from build123d import *

# Parameters (mm, degrees)
SKETCH1_W           = 141.478
SKETCH1_H           = 121.412
SKETCH1_R           = 3.175
SKETCH1_W_2         = 98.298
SKETCH1_H_2         = 38.862
BOSS_EXTRUDE1_DEPTH = 6.35
SKETCH2_W           = 61.473578211
SKETCH2_H           = 35.56
CUT_EXTRUDE1_DEPTH  = 3.81
SKETCH3_R           = 1.143
CUT_EXTRUDE2_DEPTH  = 158.770193915
SKETCH4_R           = 1.905
CUT_EXTRUDE3_DEPTH  = 158.770193915


with BuildPart() as part:
    # Sketch1 → Boss-Extrude1 (new body)
    with BuildSketch(Plane.XY):
        with Locations((49.149, 41.656)):
            Rectangle(SKETCH1_W, SKETCH1_H)
        with Locations((98.298, 80.772)):
            Circle(SKETCH1_R, mode=Mode.SUBTRACT)
        with Locations((49.149, 19.431)):
            Rectangle(SKETCH1_W_2, SKETCH1_H_2, mode=Mode.SUBTRACT)
    extrude(amount=BOSS_EXTRUDE1_DEPTH)

    # Sketch2 → Cut-Extrude1 (cut)
    with BuildSketch(Plane(origin=(0, 0, 0), x_dir=(-1, 0, 0), z_dir=(0, 0, -1))):
        with Locations((-30.736789106, 56.642)):
            Rectangle(SKETCH2_W, SKETCH2_H)
    extrude(amount=-CUT_EXTRUDE1_DEPTH, mode=Mode.SUBTRACT)

    # Sketch3 → Cut-Extrude2 (cut, through all)
    with BuildSketch(Plane.XY.offset(6.35)):
        with Locations((2.6416, 46.9138)):
            Circle(SKETCH3_R)
        with Locations((95.6564, 46.9138)):
            Circle(SKETCH3_R)
        with Locations((95.6564, -8.0518)):
            Circle(SKETCH3_R)
        with Locations((2.6416, -8.0518)):
            Circle(SKETCH3_R)
    extrude(amount=-CUT_EXTRUDE2_DEPTH, mode=Mode.SUBTRACT)

    # Sketch4 → Cut-Extrude3 (cut, through all)
    with BuildSketch(Plane.XY.offset(6.35)):
        with Locations((-16.51, 97.282)):
            Circle(SKETCH4_R)
        with Locations((-16.51, -13.97)):
            Circle(SKETCH4_R)
        with Locations((114.808, -13.97)):
            Circle(SKETCH4_R)
        with Locations((114.808, 97.282)):
            Circle(SKETCH4_R)
    extrude(amount=-CUT_EXTRUDE3_DEPTH, mode=Mode.SUBTRACT)


solid = part.part
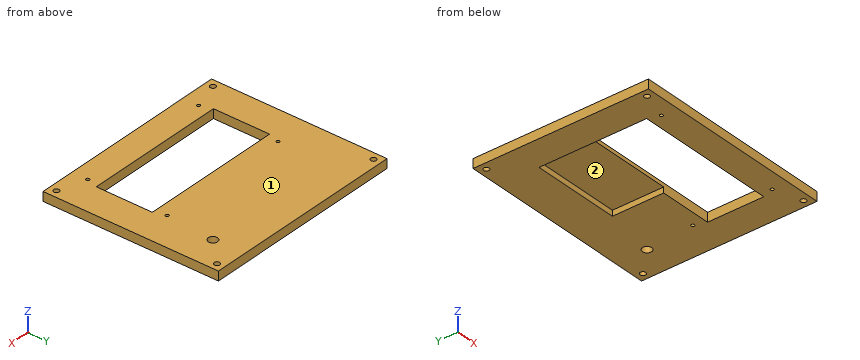
Geometry check sheet. Reference: the model listing, model coordinates, mm. Face numbers are marked on the shaded views. Round coordinates to 2 decimals unless told otherwise and drop trailing zeros. Order: outer loops, then holes, each group sorted by start corner. A loop starts at its lowest first (then second) coordinate and runs counter-clockwise, first axis right, second up. Notation, with made-up numbers: M -38,16.5 L -7,16.5 A19 cw -7,31.5 Z; hole C -32.75,83 d10. An arc over 180 degrees is marked long. Write each question's results on one line, items separated by ' | '. Start each with the question number.
1. Cross-section at B-B on x = 11. Record the boundary of the cut face in (y, z).
2. Cross-section at C-C on y = -13.97. Record the boundary of the cut face in (x, z) (3 decimals), plus the area to 3 significant figures.
3. Go/stop test with flat-tipped pins: P1, Ø5, axis at x = 47, y = 4, coming from the +Z side; P2, Ø18, axis at x = 41, y = 58, coming from the -Z side. Record where each tip stops, or that it passes through.
4. Cross-section at A-A on y = 6.5. Record the boundary of the cut face in (x, z), plus the area to 3 significant figures.
5. Cross-section at D-D on x = -16.51. Record the boundary of the cut face in (y, z) (3 decimals).
6. Material ranges on L1, parallel to Y at x = -16.51, z = 1.75 (3 decimals); L2, parallel to X at y = 39, z = 1.5; L3, parallel to Y at x = 47, z = 2.5, recorded low to high. Write a range as from..to.
7. Draft check along Y on the marked faces 1 and 2. Enter one of: pulls with the +Y half, pulls with the -Y half, needs draft (parallel to the pull), parting line crosses it, or undercut.
Resolved:
1) outline: M -19.05,0 L 0,0 L 0,6.35 L -19.05,6.35 Z; M 38.86,3.81 L 74.42,3.81 L 74.42,0 L 102.36,0 L 102.36,6.35 L 38.86,6.35 Z
2) outline: M -21.59,0 L -18.415,0 L -18.415,6.35 L -21.59,6.35 Z; M -14.605,0 L 112.903,0 L 112.903,6.35 L -14.605,6.35 Z; M 116.713,0 L 119.888,0 L 119.888,6.35 L 116.713,6.35 Z | area: 850 mm2
3) P1: through | P2: z = 3.81
4) outline: M -21.59,0 L 0,0 L 0,6.35 L -21.59,6.35 Z; M 98.3,0 L 119.89,0 L 119.89,6.35 L 98.3,6.35 Z | area: 274 mm2
5) outline: M -19.05,0 L -15.875,0 L -15.875,6.35 L -19.05,6.35 Z; M -12.065,0 L 95.377,0 L 95.377,6.35 L -12.065,6.35 Z; M 99.187,0 L 102.362,0 L 102.362,6.35 L 99.187,6.35 Z
6) L1: -19.05..-15.875, -12.065..95.377, 99.187..102.362 | L2: -21.59..0, 61.47..119.89 | L3: -19.05..0, 74.42..102.36
7) face 1: needs draft | face 2: undercut
